```python
from build123d import *

# Parameters (mm, degrees)
F1_DEPTH  = 25.4
F3_DEPTH  = 25.4
F5_DEPTH  = 25.4
F7_DEPTH  = 5.08
F10_DEPTH = 5.08
F11_DEPTH = 5.08


with BuildPart() as f1:
    # F0 (on Right) → F1 (new body)
    with BuildSketch(Plane.YZ):
        Polygon((59.1682344675, -36.3681837916), (49.3768006563, -8.6724124849), (7.9730236903, -8.6724124849), (-2.9374300502, 8.9521678165), (-38.4663492441, 8.9521678165), (-48.2577830553, 21.5411558747), (-72.8762373328, 21.5411558747), (-72.8762373328, -30.4933227599), (-72.8762373328, -36.3681837916), align=None)
    extrude(amount=F1_DEPTH)

    # F2 (on Right) → F3 (cut)
    with BuildSketch(Plane.YZ):
        Polygon((-51.3350889087, 17.6245812327), (-67.5608962774, 17.3448249698), (-67.5608962774, -31.8920984864), (51.6148433089, -31.8920984864), (45.1804734766, -13.4282521904), (5.4552280344, -13.4282521904), (-6.2944926322, 5.0355945714), (-42.103163898, 5.0355945714), align=None)
    extrude(amount=-F3_DEPTH, mode=Mode.SUBTRACT)

    # F4 (on face) → F5 (cut)
    with BuildSketch(Plane.YZ.offset(25.4)):
        Polygon((-51.6148433089, 17.3448249698), (-69.5191770792, 17.3448249698), (-69.5191770792, -32.1718528867), (53.0136227608, -32.1718528867), (46.0203764525, -12.3909551978), (4.0564518422, -12.3909551978), (-6.574248895, 5.0355945714), (-42.3829182982, 5.0355945714), align=None)
    extrude(amount=-F5_DEPTH, mode=Mode.SUBTRACT)

    # F6 (on Right) → F7 (join)
    with BuildSketch(Plane.YZ):
        Polygon((53.0136190355, -31.6123440862), (45.7399822772, -12.5889861956), (4.3362067081, -12.8687405959), (-6.0147377662, 4.1963290423), (-42.1031676233, 4.1963290423), (-51.3350889087, 16.5055599064), (-68.9596682787, 16.5055599064), (-68.4001594782, -31.6123440862), align=None)
    extrude(amount=F7_DEPTH)

    # F8 (on Right) → F10 (join)
    with BuildSketch(Plane.YZ):
        Polygon((5.4552271031, -11.7497202009), (-7.4135139585, 4.7558392398), (-42.1031676233, 4.7558392398), (-50.7755763829, 17.0650705695), (-69.7989314795, 17.0650705695), (-69.7989314795, -30.213566497), (-69.7989314795, -32.1718528867), (53.0136190355, -32.1718528867), (46.8590036035, -11.7497202009), align=None)
    extrude(amount=F10_DEPTH)

    # F9 (on Right) → F11 (join)
    with BuildSketch(Plane.YZ):
        Polygon((56.2891028821, -33.4541499615), (49.1134338081, -13.0950817838), (49.1134338081, -10.6687908992), (7.4033048004, -10.6687908992), (-4.491108004, 6.529154256), (-40.5934713781, 6.529154256), (-49.6454611421, 18.8511218876), (-70.4428181052, 18.8511218876), (-70.4428181052, -33.4541499615), align=None)
    extrude(amount=F11_DEPTH)


solid = f1.part
```
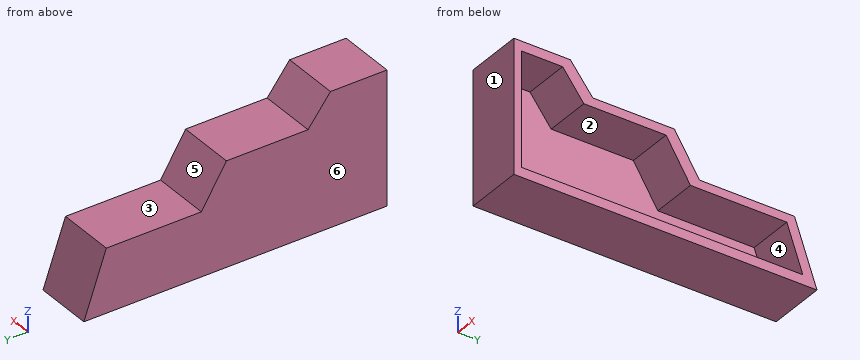
Build history of the part. All positions in model axes, mm. Face numbers are marked on the shaded views. A direction names the side the tool comes from. Coordinates: 2 decimals unless noted, no trailing zeros. Order: outer loops, then holes, each group sorted by start corner. A loop starts at its lowest first (then second) coordinate and runs counter-clockwise, first axis right, second up. Notation, with made-up numbers: (-4.75, 80) -> (33.25, 80) arc R13 ccw to (33.25, 84) -> close; hole circle Ø9 at (53, 28). An arc over 180 degrees is marked (long way). Answer in a Markdown table with one row per item. Add a question column.
Q1. Which spindle directions (+Z, -Z, +X, -X, +Y, -Y) get a long thin tool onto all of the face, cutting with end or side? Do the marked faces 1, 2 and 3. Say none if no direction does.
Q2. Band-saw the part on A-A, the plane y = 43. List the corners of the cut face in (x, z).
Q3. Band-saw the part on B-B, the plane x = 21.75. List the corners of the cut face in (y, z), then the cut area to 3 significant figures.
Q4. Drop flat-ended pins along their axis: pin 1 (1 mm diameter, centred on y = 18.5, z = -23.5, fed in from +X); pin 2 (12.5 mm diameter, centred on x = 8.5, y = 31.5, fed in from +Z); pin 3 (10 mm diameter, centred on x = 13, y = 2.5, fed in from +Z). Give the stop position or say it passes through.
Q5. Mould opens along Y. For the marked faces 4, 5 and 6 say: +Y half, -Y half, draft (parallel to the pull), parting line (faces both ways), or undercut.
Q6. Band-saw the part on C-C, the plane z = -7. List the corners of the cut face in (x, y).
Q7. Wall check: line 1 along Z through (x, y) = (19, 25.5); line 2 along Z through (x, y) = (11.75, -61); line 3 along Y through (x, z) = (17, -1.5). Give the ranges that are in metal, low to high. Write a range as [from, to].
Answers follow:
| question | item | result |
|---|---|---|
| 1 | face 1 | +Z, -Z, +X, -X, -Y |
| 1 | face 2 | +X |
| 1 | face 3 | +Z, +X, -X, +Y |
| 2 | outline | (0, -36.37) -> (25.4, -36.37) -> (25.4, -32.17) -> (5.08, -32.17) -> (5.08, -12.39) -> (25.4, -12.39) -> (25.4, -8.67) -> (0, -8.67) -> close |
| 3 | outline | (-72.88, -36.37) -> (59.17, -36.37) -> (49.38, -8.67) -> (7.97, -8.67) -> (-2.94, 8.95) -> (-38.47, 8.95) -> (-48.26, 21.54) -> (-72.88, 21.54) -> close; hole (-69.52, -32.17) -> (53.01, -32.17) -> (46.02, -12.39) -> (4.06, -12.39) -> (-6.57, 5.04) -> (-42.38, 5.04) -> (-51.61, 17.34) -> (-69.52, 17.34) -> close |
| 3 | area | 1,400 mm^2 |
| 4 | pin 1 | x = 5.08 |
| 4 | pin 2 | z = -8.67 |
| 4 | pin 3 | z = 8.25 |
| 5 | face 4 | undercut |
| 5 | face 5 | +Y half |
| 5 | face 6 | draft |
| 6 | outline | (0, -72.88) -> (25.4, -72.88) -> (25.4, -69.52) -> (5.08, -69.52) -> (5.08, 0.77) -> (25.4, 0.77) -> (25.4, 6.94) -> (0, 6.94) -> close |
| 7 | line 1 | [-36.37, -32.17], [-12.39, -8.67] |
| 7 | line 2 | [-36.37, -32.17], [17.34, 21.54] |
| 7 | line 3 | [-72.88, -69.52], [-2.59, 3.53] |
